Verification items for this drawing (mm, ordinates from the low corner). Round coordinates to 2 decimals unless told otherwise and drop trailing zeros. Loops run counter-clockwise (first coordinate to the right, second up) from the corner with the lowest first, then second, coordinate; pieces in that order, holes last. Notation, with made-up numbers: (-26.75, 61) -> (-21.75, 61) arc R28 ccw to (-21.75, 83) -> close; hole circle Ø6 at (16.25, 73.5). An arc over 180 degrees is marked (long way). Use a Markdown table: item, result. Add a question column.
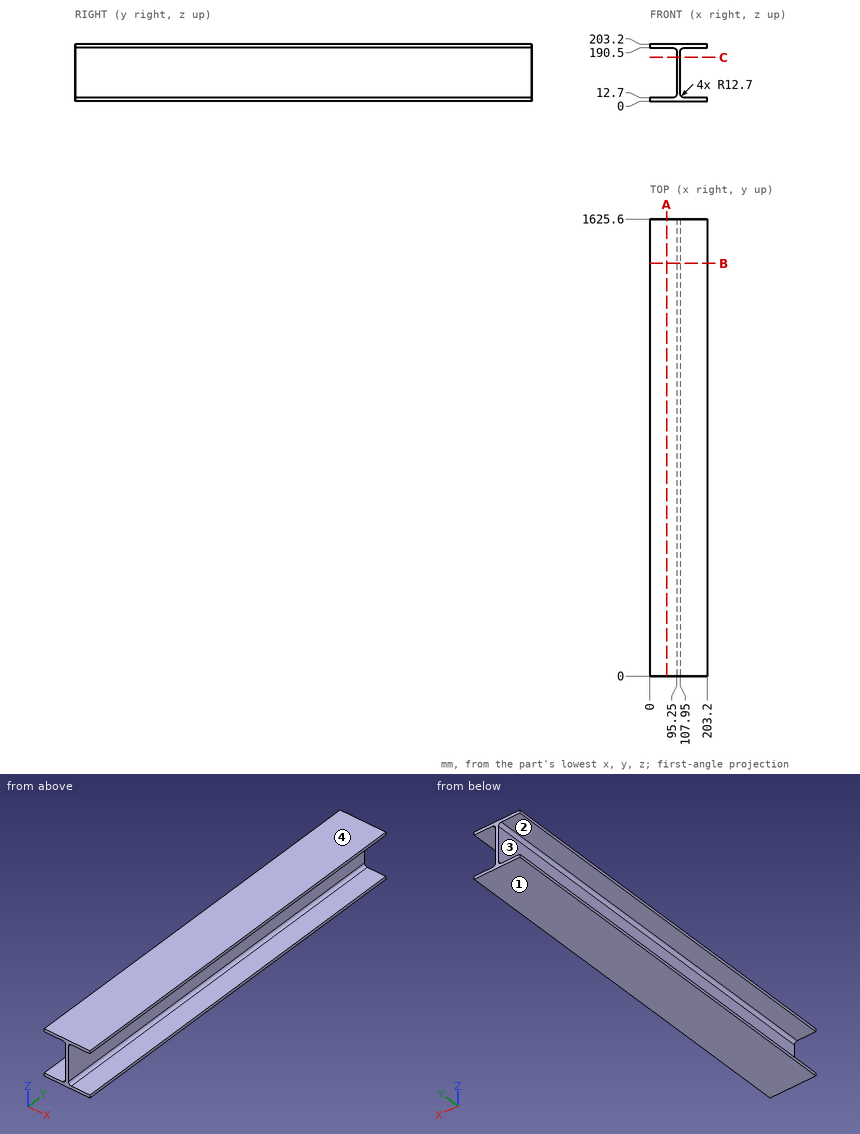
1) Go/stop test with flat-tipped pins: pin 1 (2 mm diameter, centred on x = 162, y = 194.5, fed in from -Z); pin 2 (8 mm diameter, centred on y = 997, z = 95, fed in from -X); pin 3 (10 mm diameter, centred on y = 200.5, z = 34, fed in from +X). Record where each tip stops, or that it passes through.
2) Release check for a two-part mould opening along Z. For the marked faces 1, 2, 3 and 4 record: released by +Z, released by -Z, zero draft, split by the parting line, or undercut.
3) Thickness scan on line 1 (Z direction, x = 153.5, y = 142.5); line 2 (Z direction, x = 84, y = 97); line 3 (X direction, y = 138.5, z = 148.5). Record the ranges inside material, lowest first.
4) Sectioned sample at A-A on x = 59.5. Enter the section's corners in (y, z).
5) Sectioned sample at C-C on z = 156. Enter the section's corners in (x, y).
6) Sectioned sample at B-B on y = 1468.5. Enter the section's corners in (x, z).
Geometry results:
| question | item | result |
|---|---|---|
| 1 | pin 1 | z = 0 |
| 1 | pin 2 | x = 95.25 |
| 1 | pin 3 | x = 107.95 |
| 2 | face 1 | released by -Z |
| 2 | face 2 | undercut |
| 2 | face 3 | undercut |
| 2 | face 4 | released by +Z |
| 3 | line 1 | 0 to 12.7, 190.5 to 203.2 |
| 3 | line 2 | 0 to 12.78, 190.42 to 203.2 |
| 3 | line 3 | 95.25 to 107.95 |
| 4 | outline | (0, 0) -> (1625.6, 0) -> (1625.6, 12.7) -> (0, 12.7) -> close; (0, 190.5) -> (1625.6, 190.5) -> (1625.6, 203.2) -> (0, 203.2) -> close |
| 5 | outline | (95.25, 0) -> (107.95, 0) -> (107.95, 1625.6) -> (95.25, 1625.6) -> close |
| 6 | outline | (0, 0) -> (203.2, 0) -> (203.2, 12.7) -> (120.65, 12.7) arc R12.7 cw to (107.95, 25.4) -> (107.95, 177.8) arc R12.7 cw to (120.65, 190.5) -> (203.2, 190.5) -> (203.2, 203.2) -> (0, 203.2) -> (0, 190.5) -> (82.55, 190.5) arc R12.7 cw to (95.25, 177.8) -> (95.25, 25.4) arc R12.7 cw to (82.55, 12.7) -> (0, 12.7) -> close |
